from build123d import *

# Parameters (mm, degrees)
BOSS_EXTRUDE1_DEPTH     = 25.4
F_6_CLEARANCE_HOLE1_D   = 3.7973
F_1_4_CLEARANCE_HOLE1_D = 6.7564
BOSS_EXTRUDE2_DEPTH     = 3.048
BOSS_EXTRUDE3_DEPTH     = 3.048
FILLET1_R               = 1.27
CHAMFER1_SIZE           = 6.35


with BuildPart() as part:
    # Sketch1 → Boss-Extrude1 (new body)
    with BuildSketch(Plane.XY):
        Polygon((0, 0), (0, 25.4), (3.81, 25.4), (3.81, 3.81), (31.75, 3.81), (31.75, 0), align=None)
    extrude(amount=BOSS_EXTRUDE1_DEPTH)

    # #6 Clearance Hole1 (through all)
    with Locations(Plane(origin=(0, 3.81, 0), x_dir=(1, 0, 0), z_dir=(0, 1, 0))):
        with Locations((10.2108, -12.7), (25.2222, -12.7)):
            Hole(F_6_CLEARANCE_HOLE1_D / 2)

    # 1/4 Clearance Hole1 (through all)
    with Locations(Plane(origin=(3.81, 0, 0), x_dir=(0, 0, -1), z_dir=(1, 0, 0))):
        with Locations((-12.7, 16.51)):
            Hole(F_1_4_CLEARANCE_HOLE1_D / 2)

    # Sketch6 → Boss-Extrude2 (add)
    with BuildSketch(Plane.XY.offset(25.4)):
        Polygon((3.81, 3.81), (17.78, 3.81), (3.81, 14.605), align=None)
    extrude(amount=-BOSS_EXTRUDE2_DEPTH)

    # Sketch7 → Boss-Extrude3 (add)
    with BuildSketch(Plane(origin=(0, 0, 0), x_dir=(-1, 0, 0), z_dir=(0, 0, -1))):
        Polygon((-3.81, 3.81), (-17.78, 3.81), (-3.81, 14.605), align=None)
    extrude(amount=-BOSS_EXTRUDE3_DEPTH)

    # Fillet1
    fillet1_edges = [part.edges().sort_by_distance(p)[0] for p in [
        (3.81, 3.81, 12.7),
        (3.81, 9.2075, 22.352),
        (3.81, 14.605, 23.876),
        (10.795, 3.81, 22.352),
        (17.78, 3.81, 23.876),
        (3.81, 9.2075, 3.048),
        (3.81, 14.605, 1.524),
        (10.795, 3.81, 3.048),
        (17.78, 3.81, 1.524),
    ]]
    fillet(fillet1_edges, radius=FILLET1_R)

    # Chamfer1
    chamfer1_edges = [part.edges().sort_by_distance(p)[0] for p in [
        (1.905, 25.4, 25.4),
        (1.905, 25.4, 0),
        (31.75, 1.905, 0),
        (31.75, 1.905, 25.4),
    ]]
    chamfer(chamfer1_edges, length=CHAMFER1_SIZE)


solid = part.part
Input: part model. Units: mm. Frame: model coordinates. A direction names the side the tool comes from. Coordinates: 2 decimals unless noted, no trailing zeros. Order: outer loops, then holes, each group sorted by start corner. A loop starts at its lowest first (then second) coordinate and runs counter-clockwise, first axis right, second up. Notation, with made-up numbers: M 66,58.25 L 90,58.25 A20 ccw 90,81.25 Z; hole C 26.25,-37 d2. An arc over 180 degrees is marked long. One line per question, with ' | ' between items.
Item 1: Draft query along Z for faces 1 (the flat face through (28.5, 1.9, 22.3)), 2 (the flat face through (18, 3.81, 13)), 3 (the flat face through (28.6, 1.9, 3.2)). Return one class per face: released by +Z, released by -Z, zero draft, split by the parting line, or undercut.
Geometry results:
face 1: released by +Z | face 2: undercut | face 3: released by -Z
Item 2: Ray query, line 1 along X through (y, z) = (1.5, 12.7); line 2 along Z through (x, y) = (6, 11); line 3 along Y through (x, z) = (0.9, 12.7). Return the intervals inside material, ascending.
Geometry results:
line 1: x = 0 to 8.31, 12.11 to 23.32, 27.12 to 31.75 | line 2: z = 0 to 3.05, 22.35 to 25.4 | line 3: y = 0 to 13.13, 19.89 to 25.4
Item 3: Section A-A (y = 16.51). Output: boundary loops of the cut face in (x, z).
Geometry results:
outline: M 0,0 L 3.81,0 L 3.81,9.32 L 0,9.32 Z; M 0,16.08 L 3.81,16.08 L 3.81,25.4 L 0,25.4 Z
Item 4: Pin query (flat end, axial travel): pin 1 (6 mm diameter, centred on x = 25.22, z = 12.7, fed in from +Y); pin 2 (2 mm diameter, centred on y = 22, z = 21, fed in from +X). Return the tip coordinate at first contact, or that it passes through.
Geometry results:
pin 1: stops at y = 3.81 | pin 2: stops at x = 3.81
Item 5: Section C-C (x = 10). Output: boundary loops of the cut face in (y, z), then the cut area to 3 significant figures.
Geometry results:
outline: M 0,0 L 9.82,0 L 9.82,3.05 L 5.08,3.05 A1.27 cw 3.81,4.32 L 3.81,10.81 L 0,10.81 Z; M 0,14.59 L 3.81,14.59 L 3.81,21.08 A1.27 cw 5.08,22.35 L 9.82,22.35 L 9.82,25.4 L 0,25.4 Z | area: 120 mm^2
Item 6: Section B-B (z = 12.7). Output: boundary loops of the cut face in (x, y).
Geometry results:
outline: M 0,0 L 8.31,0 L 8.31,3.81 L 5.08,3.81 A1.27 cw 3.81,5.08 L 3.81,13.13 L 0,13.13 Z; M 0,19.89 L 3.81,19.89 L 3.81,25.4 L 0,25.4 Z; M 12.11,0 L 23.32,0 L 23.32,3.81 L 12.11,3.81 Z; M 27.12,0 L 31.75,0 L 31.75,3.81 L 27.12,3.81 Z
Item 7: Reachability of faces 4 (the flat face through (3.81, 13, 15)), 5 (the flat face through (10, 5, 25.4)) from +Z, -Z, +X, -X, +Y, -Y: full face, straight path, thin tool, end or side. Return the list, or none.
Geometry results:
face 4: +X, +Y | face 5: +Z, +X, -X, +Y, -Y
Item 8: Section D-D (z = 8.25). Output: boundary loops of the cut face in (x, y).
Geometry results:
outline: M 0,0 L 31.75,0 L 31.75,3.81 L 5.08,3.81 A1.27 cw 3.81,5.08 L 3.81,25.4 L 0,25.4 Z
